For this review, take the finished solid that the model builds, in its own axes (mm). A direction names the side the tool comes from. Coordinates: 2 decimals unless noted, no trailing zeros. Write each loop counter-clockwise with the first axis right and the second up, starting at its lowest first coordinate (ties: lowest second). Pieces come first, ordered by that corner, then holes. Notation, with made-up numbers: (8.5, 15) - (15.5, 15) arc R19 ccw to (15.5, 31) - close; hole circle Ø5 at (71.25, -24). An arc over 180 degrees is marked (long way). Write each question's results on one line, items separated by ' | '.
from build123d import *

# Parameters (mm, degrees)
SKETCH1_W           = 17.78
SKETCH1_H           = 17.78
BOSS_EXTRUDE1_DEPTH = 17.78
FILLET1_R           = 2.54
SKETCH2_R           = 1.574444288
BOSS_EXTRUDE2_DEPTH = 7.62


with BuildPart() as part:
    # Sketch1 → Boss-Extrude1 (new body)
    with BuildSketch(Plane.XY):
        Rectangle(SKETCH1_W, SKETCH1_H)
    extrude(amount=BOSS_EXTRUDE1_DEPTH)

    # Fillet1
    fillet1_edges = [part.edges().sort_by_distance(p)[0] for p in [
        (8.89, -8.89, 8.89),
        (-8.89, -8.89, 8.89),
        (-8.89, 8.89, 8.89),
        (8.89, 8.89, 8.89),
    ]]
    fillet(fillet1_edges, radius=FILLET1_R)

    # Sketch2 → Boss-Extrude2 (add)
    with BuildSketch(Plane(origin=(0, 0, 0), x_dir=(-1, 0, 0), z_dir=(0, 0, -1))):
        Circle(SKETCH2_R)
    extrude(amount=BOSS_EXTRUDE2_DEPTH)


solid = part.part
Q1. For faces 4 (the face through (0, 0, -7.62)), 5 (the face through (0.2, 1.56, -3.76)), list the 3-axis set-ups (+Z, -Z, +X, -X, +Y, -Y) from which the entire face can be reached by the end or side of a thin tool; tool diameter is ignored.
Results found:
face 4: -Z, +X, -X, +Y, -Y | face 5: -Z
Q2. Take a section at C-C on y = 5.25. State the section outline as (x, z) points.
Results found:
outline: (-8.89, 0) - (8.89, 0) - (8.89, 17.78) - (-8.89, 17.78) - close
Q3. Take a section at A-A on z = 14. State the section outline as (x, y) points.
Results found:
outline: (-8.89, -6.35) arc R2.54 ccw to (-6.35, -8.89) - (6.35, -8.89) arc R2.54 ccw to (8.89, -6.35) - (8.89, 6.35) arc R2.54 ccw to (6.35, 8.89) - (-6.35, 8.89) arc R2.54 ccw to (-8.89, 6.35) - close
Q4. For pin 1 (6 mm diameter, centred on x = -3.5, y = -6, fed in from -Z); pin 2 (2 mm diameter, centred on x = -6, z = -2, fed in from -Y), all flat-tipped, find the tip position at first contact; note any pin that passes through.
Results found:
pin 1: z = 0 | pin 2: through
Q5. Mouldability with a two-part tool opening along X and no side actions: class faces 1 (the face through (-8.166, 8.126, 9.014)), 2 (the face through (8.89, 0, 9)), 3 (the face through (0, 0, 17.78)) as pulls with the +X half, pulls with the -X half, needs draft (parallel to the pull), parting line crosses it, or undercut.
Results found:
face 1: pulls with the -X half | face 2: pulls with the +X half | face 3: needs draft
Q6. Wall thickness on line 1 along Z through (x, y) = (-8, -8); line 2 along Y through (x, z) = (0, -1); line 3 along X through (y, z) = (-6.5, 7.75): over which ranges is each line inside the solid? List them lowest first. Write a range as from..to.
Results found:
line 1: 0..17.78 | line 2: -1.57..1.57 | line 3: -8.89..8.89
Q7. Take a section at B-B on x = 0. State the section outline as (y, z) points, plus the area to 3 significant figures.
Results found:
outline: (-8.89, 0) - (-1.57, 0) - (-1.57, -7.62) - (1.57, -7.62) - (1.57, 0) - (8.89, 0) - (8.89, 17.78) - (-8.89, 17.78) - close | area: 340 mm2
